```python
from build123d import *

# Parameters (mm, degrees)
F0_W     = 12.7
F0_H     = 3.175
F0_W_2   = 3.175
F0_H_2   = 12.7
F1_DEPTH = 3.175


# Not quite as in the source:
# - a feature names something its author has since deleted; it is built from what else it names


with BuildPart() as f1:
    # F0 (on Front) → F1 (new body)
    with BuildSketch(Plane.XZ):
        Polygon((15.7950905681, 13.6112950251), (-104.8549094319, 13.6112950251), (-104.8549094319, 7.2612950251), (-104.8549094319, -5.4387049749), (-104.8549094319, -11.7887049749), (-101.6799094319, -11.7887049749), (-88.9799094319, -11.7887049749), (-76.2799094319, -11.7887049749), (-63.5799094319, -11.7887049749), (-50.8799094319, -11.7887049749), (-38.1799094319, -11.7887049749), (-25.4799094319, -11.7887049749), (-12.7799094319, -11.7887049749), (-0.0799094319, -11.7887049749), (12.6200905681, -11.7887049749), (15.7950905681, -11.7887049749), (15.7950905681, -5.4387049749), (15.7950905681, 7.2612950251), align=None)
        with Locations((-44.5299094319, -13.3762049749)):
            Rectangle(F0_W, F0_H)
        with Locations((-19.1299094319, -13.3762049749)):
            Rectangle(F0_W, F0_H)
        with Locations((-95.3299094319, -13.3762049749)):
            Rectangle(F0_W, F0_H)
        with Locations((-69.9299094319, -13.3762049749)):
            Rectangle(F0_W, F0_H)
        with Locations((6.2700905681, -13.3762049749)):
            Rectangle(F0_W, F0_H)
        with Locations((-106.4424094319, 0.9112950251)):
            Rectangle(F0_W_2, F0_H_2)
        with Locations((17.3825905681, 0.9112950251)):
            Rectangle(F0_W_2, F0_H_2)
    extrude(amount=F1_DEPTH)


solid = f1.part
```
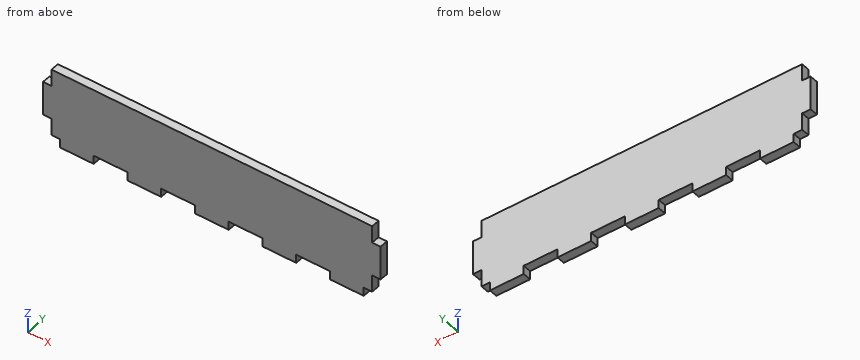
Work out the finished part from the listing and answer in its coordinate system (mm). Coordinates: 2 decimals unless noted, no trailing zeros. Loops run counter-clockwise (first coordinate to the right, second up) from the corner with the lowest first, then second, coordinate; pieces in that order, holes last. Notation, with made-up numbers: (56, 62) -> (60, 62) arc R31 ccw to (60, 90) -> close; hole circle Ø9 at (34.25, 23.25). An arc over 180 degrees is marked (long way). Answer as CSV lines item,"result".
Q1. Find the intervals of material crossed by probe 1 along X at (y, z) = (-1.3, -13.5); probe 2 along Z at (x, y) = (-7, -2.6); probe 3 along X at (y, z) = (-0.35, -10.25), in increasing order.
Findings:
probe 1,"x = -101.68 to -88.98, -76.28 to -63.58, -50.88 to -38.18, -25.48 to -12.78, -0.08 to 12.62"
probe 2,"z = -11.79 to 13.61"
probe 3,"x = -104.85 to 15.8"
Q2. Each of these flat-tipped pins is pushed along its axis until it touches: pin 1 (1.6 mm diameter, centred on x = -103, y = -2, fed in from -Z); pin 2 (1 mm diameter, centred on y = -1, z = -8, fed in from +X); pin 3 (1.6 mm diameter, centred on y = -1, z = -14, fed in from -X). Where does it stop, or does it pass through?
Findings:
pin 1,"stops at z = -11.79"
pin 2,"stops at x = 15.8"
pin 3,"stops at x = -101.68"
Q3. The part is cut by section C-C on x = -27. Write down the section's boundary in (y, z) (3 decimals).
Findings:
outline,"(-3.175, -11.789) -> (0, -11.789) -> (0, 13.611) -> (-3.175, 13.611) -> close"
Q4. The part is cut by section B-B on z = 10. Write down the section's boundary in (x, y) (3 decimals), and give its area (3 significant figures).
Findings:
outline,"(-104.855, -3.175) -> (15.795, -3.175) -> (15.795, 0) -> (-104.855, 0) -> close"
area,"383 mm²"
